Input: part model. Units: mm. Frame: model coordinates. A direction names the side the tool comes from. Give positions to 0.01 mm unless a question says otherwise; leave off trailing zeros. Loops run counter-clockwise (first coordinate to the right, second up) from the corner with the lowest first, then second, coordinate; pieces in that order, holes last.
from build123d import *

# Parameters (mm, degrees)
F1_DEPTH = 3.5


with BuildPart() as f1:
    # F0 (on Top) → F1 (new body)
    with BuildSketch(Plane.XY):
        with BuildLine():
            ThreePointArc((-3.729947, 2.517439), (-4.52425, 2.077468), (-5.347059, 2.461496))
            ThreePointArc((-5.347059, 2.461496), (-9.812645, 3.778487), (-12.499931, -0.023411))
            ThreePointArc((-12.499931, -0.023411), (-9.244431, -3.930117), (-4.785714, -1.484615))
            ThreePointArc((-4.785714, -1.484615), (-4.774576, -1.144209), (-4.984035, -0.875644))
            ThreePointArc((-4.984035, -0.875644), (-5.404829, -0.823614), (-5.714286, -1.113461))
            ThreePointArc((-5.714286, -1.113461), (-9.03795, -2.951374), (-11.49942, -0.058999))
            ThreePointArc((-11.49942, -0.058999), (-9.504036, 2.826997), (-6.135294, 1.846122))
            ThreePointArc((-6.135294, 1.846122), (-4.489676, 1.078066), (-2.90107, 1.958008))
            ThreePointArc((-2.90107, 1.958008), (1.001067, 3.353784), (3.499678, 0.047456))
            ThreePointArc((3.499678, 0.047456), (0.787879, -3.410168), (-3.165812, -1.492527))
            ThreePointArc((-3.165812, -1.492527), (-3.582024, -1.207046), (-4.034966, -1.429704))
            ThreePointArc((-4.034966, -1.429704), (-4.888074, -3.648968), (-4.724786, -6.020942))
            ThreePointArc((-4.724786, -6.020942), (-4.462085, -6.330099), (-4.056583, -6.342665))
            ThreePointArc((-4.056583, -6.342665), (-3.794678, -6.096503), (-3.765574, -5.738253))
            ThreePointArc((-3.765574, -5.738253), (-3.948415, -4.386443), (-3.717805, -3.041958))
            ThreePointArc((-3.717805, -3.041958), (-3.567792, -2.909236), (-3.377955, -2.973117))
            ThreePointArc((-3.377955, -2.973117), (1.588529, -4.210294), (4.5, -0.000792))
            ThreePointArc((4.5, -0.000792), (1.316669, 4.303067), (-3.729947, 2.517439))
        make_face()
    extrude(amount=F1_DEPTH)


solid = f1.part
(1) Reachability of faces 1 (the cylindrical face through (-3.95, -4.41, 1.73)), 2 (the flat face through (-5.3, -1.3, 0)) from +Z, -Z, +X, -X, +Y, -Y: full face, straight path, thin tool, end or side. Return the list, or none.
Values follow:
face 1: +Z, -Z
face 2: -Z, +X, -X, +Y, -Y
(2) Ray query, probe 1 along X at (y, z) = (-2.75, 3); probe 2 along X at (y, z) = (0, 0.9); probe 3 along X at (y, z) = (2.25, 2.6). Return the intervals inside material, ascending.
Values follow:
probe 1: x = -11.4 to -9.7, -7.3 to -5.6, -4.67 to -2.17, 2.17 to 3.56
probe 2: x = -12.5 to -11.5, 3.5 to 4.5
probe 3: x = -11.81 to -10.48, -6.52 to -5.12, -4 to -2.68, 2.68 to 3.9
(3) Cut plane A-A (x = -10). Return the cut outline in (y, z), and give its area (3 significant figures).
Values follow:
outline: (-3.71, 0) - (-2.6, 0) - (-2.6, 3.5) - (-3.71, 3.5) - close; (2.6, 0) - (3.71, 0) - (3.71, 3.5) - (2.6, 3.5) - close
area: 7.77 mm2
(4) Cut plane B-B (y = 2.25). Return the cut outline in (x, z), and give its area (3 significant figures).
Values follow:
outline: (-11.81, 0) - (-10.48, 0) - (-10.48, 3.5) - (-11.81, 3.5) - close; (-6.52, 0) - (-5.12, 0) - (-5.12, 3.5) - (-6.52, 3.5) - close; (-4, 0) - (-2.68, 0) - (-2.68, 3.5) - (-4, 3.5) - close; (2.68, 0) - (3.9, 0) - (3.9, 3.5) - (2.68, 3.5) - close
area: 18.4 mm2
(5) Cut plane D-D (z = 1.1). Return the cut outline in (x, y).
Values follow:
outline: (-6.14, 1.85) arc R2 ccw to (-2.9, 1.96) arc R3.5 cw (long way) to (-3.17, -1.49) arc R0.5 ccw to (-4.03, -1.43) arc R5.5 ccw to (-4.72, -6.02) arc R0.5 ccw to (-4.06, -6.34) arc R0.5 ccw to (-3.77, -5.74) arc R4.5 cw to (-3.72, -3.04) arc R0.2 cw to (-3.38, -2.97) arc R4.5 ccw (long way) to (-3.73, 2.52) arc R1 cw to (-5.35, 2.46) arc R4 ccw (long way) to (-4.79, -1.48) arc R0.5 ccw to (-5.71, -1.11) arc R3 cw (long way) to start
(6) Pin query (flat end, axial travel): pin 1 Ø2 at (y, z) = (3.5, 1.5) entering from -X; pin 2 Ø1 at (x, z) = (2.5, 0.5) entering from -Y; pin 3 Ø1.5 at (y, z) = (-1, 3) entering from -X. Return the tip coordinate at first contact, or that it passes through.
Values follow:
pin 1: stops at x = -11.62
pin 2: stops at y = -4.03
pin 3: stops at x = -12.49
(7) Mould query, pull axis Y, two halves, no side actions, for faces 3 (the cylindrical face through (-3.57, -1.21, 1.73)), 4 (the cylindrical face through (-4.883, -3.616, 1.726)), 5 (the flat face through (-5.3, -1.3, 3.5)), 6 (the cylindrical face through (-4.51, 2.08, 1.73)). Classes: +Y half, -Y half, draft (parallel to the pull), parting line (faces both ways), or undercut.
Values follow:
face 3: undercut
face 4: undercut
face 5: draft
face 6: +Y half
(8) Cut plane C-C (y = 3.75). Return the cut outline in (x, z), and give its area (3 significant figures).
Values follow:
outline: (-9.89, 0) - (-7.11, 0) - (-7.11, 3.5) - (-9.89, 3.5) - close; (-2.49, 0) - (2.49, 0) - (2.49, 3.5) - (-2.49, 3.5) - close
area: 27.2 mm2
